Autodesk Inventor part; units mm, degrees
ref_plane "YZ Plane" through (0, 0, 0) normal (1, 0, 0) x (0, 1, 0)
ref_plane "XZ Plane" through (0, 0, 0) normal (0, 1, 0) x (-1, 0, 0)
ref_plane "XY Plane" through (0, 0, 0) normal (0, 0, 1) x (1, 0, 0)
ref_plane "Work Plane1" through (0, 0, 0) normal (0, 0, 1) x (1, 0, 0)
sketch "Sketch1" plane through (0, 0, 0) normal (0, 0, 1) x (1, 0, 0)
  circle A0 centre (0, 52.9) radius 8
  line L0 (-75, -117.1) -> (75, -117.1)
  line L1 (75, -117.1) -> (75, 82.9)
  line L2 (75, 82.9) -> (-75, 82.9)
  line L3 (-75, 82.9) -> (-75, -117.1)
  circle A1 centre (0, -87.1) radius 8
  circle A2 centre (0, -16.8) radius 16
  line L4 (0.031, -34.3) -> (-1.6246, -39.8894)
  line L5 (-1.6246, -39.8894) -> (-3.8779, -39.222)
  line L6 (-3.8779, -39.222) -> (-3.5087, -37.9755)
  line L7 (-3.5087, -37.9755) -> (-2.8854, -38.1601)
  line L8 (-2.8854, -38.1601) -> (-1.8914, -34.8042)
  line L9 (-1.8914, -34.8042) -> (-8.2196, -32.9297)
  line L10 (-8.2196, -32.9297) -> (-9.2136, -36.2856)
  line L11 (-9.2136, -36.2856) -> (-8.5904, -36.4702)
  line L12 (-8.5904, -36.4702) -> (-8.9843, -37.8)
  line L13 (-8.9843, -37.8) -> (-15.25, -37.8)
  line L14 (-15.25, -37.8) -> (-15.25, -39.8)
  line L15 (-15.25, -39.8) -> (-17.25, -39.8)
  line L16 (-17.25, -39.8) -> (-17.25, -37.8)
  arc A3 (-21, -34.05) -> (-17.25, -37.8) centre (-17.25, -34.05) ccw
  line L17 (-21, -34.05) -> (-23, -34.05)
  line L18 (-23, -34.05) -> (-23, -32.05)
  line L19 (-23, -32.05) -> (-21, -32.05)
  line L20 (-21, -32.05) -> (-21, -26.253)
  line L21 (-21, -26.253) -> (-19.5478, -25.71)
  arc A4 (-19.5478, -25.71) -> (-20.5984, -22.9) centre (-18.6632, -23.7779) ccw
  line L22 (-20.5984, -22.9) -> (-21.4365, -23.2134)
  line L23 (-21.4365, -23.2134) -> (-22.1807, -21.2229)
  line L24 (-22.1807, -21.2229) -> (-17.3057, -19.4003)
  arc A5 (-17.5, -16.831) -> (-17.3057, -19.4003) centre (0, -16.8) ccw
  line L25 (-17.5, -16.831) -> (-23.0894, -15.1754)
  line L26 (-23.0894, -15.1754) -> (-22.422, -12.9221)
  line L27 (-22.422, -12.9221) -> (-21.1755, -13.2913)
  line L28 (-21.1755, -13.2913) -> (-21.3601, -13.9146)
  line L29 (-21.3601, -13.9146) -> (-18.0042, -14.9086)
  line L30 (-18.0042, -14.9086) -> (-16.1297, -8.5804)
  line L31 (-16.1297, -8.5804) -> (-19.4856, -7.5864)
  line L32 (-19.4856, -7.5864) -> (-19.6702, -8.2096)
  line L33 (-19.6702, -8.2096) -> (-21, -7.8157)
  line L34 (-21, -7.8157) -> (-21, -1.55)
  line L35 (-21, -1.55) -> (-23, -1.55)
  line L36 (-23, -1.55) -> (-23, 0.45)
  line L37 (-23, 0.45) -> (-21, 0.45)
  arc A6 (-17.25, 4.2) -> (-21, 0.45) centre (-17.25, 0.45) ccw
  line L38 (-17.25, 4.2) -> (-17.25, 6.2)
  line L39 (-17.25, 6.2) -> (-15.25, 6.2)
  line L40 (-15.25, 6.2) -> (-15.25, 4.2)
  line L41 (-15.25, 4.2) -> (-9.453, 4.2)
  line L42 (-9.453, 4.2) -> (-8.91, 2.7478)
  arc A7 (-8.91, 2.7478) -> (-6.1, 3.7984) centre (-6.9779, 1.8632) ccw
  line L43 (-6.1, 3.7984) -> (-6.4134, 4.6365)
  line L44 (-6.4134, 4.6365) -> (-4.4229, 5.3807)
  line L45 (-4.4229, 5.3807) -> (-2.6003, 0.5057)
  arc A8 (-0.031, 0.7) -> (-2.6003, 0.5057) centre (0, -16.8) ccw
  line L46 (-0.031, 0.7) -> (1.6246, 6.2894)
  line L47 (1.6246, 6.2894) -> (3.8779, 5.622)
  line L48 (3.8779, 5.622) -> (3.5087, 4.3755)
  line L49 (3.5087, 4.3755) -> (2.8854, 4.5601)
  line L50 (2.8854, 4.5601) -> (1.8914, 1.2042)
  line L51 (1.8914, 1.2042) -> (8.2196, -0.6703)
  line L52 (8.2196, -0.6703) -> (9.2136, 2.6856)
  line L53 (9.2136, 2.6856) -> (8.5904, 2.8702)
  line L54 (8.5904, 2.8702) -> (8.9843, 4.2)
  line L55 (8.9843, 4.2) -> (15.25, 4.2)
  line L56 (15.25, 4.2) -> (15.25, 6.2)
  line L57 (15.25, 6.2) -> (17.25, 6.2)
  line L58 (17.25, 6.2) -> (17.25, 4.2)
  arc A9 (21, 0.45) -> (17.25, 4.2) centre (17.25, 0.45) ccw
  line L59 (21, 0.45) -> (23, 0.45)
  line L60 (23, 0.45) -> (23, -1.55)
  line L61 (23, -1.55) -> (21, -1.55)
  line L62 (21, -1.55) -> (21, -7.347)
  line L63 (21, -7.347) -> (19.5478, -7.89)
  arc A10 (19.5478, -7.89) -> (20.5984, -10.7) centre (18.6632, -9.8221) ccw
  line L64 (20.5984, -10.7) -> (21.4365, -10.3866)
  line L65 (21.4365, -10.3866) -> (22.1807, -12.3771)
  line L66 (22.1807, -12.3771) -> (17.3057, -14.1997)
  arc A11 (17.5, -16.769) -> (17.3057, -14.1997) centre (0, -16.8) ccw
  line L67 (17.5, -16.769) -> (23.0894, -18.4246)
  line L68 (23.0894, -18.4246) -> (22.422, -20.6779)
  line L69 (22.422, -20.6779) -> (21.1755, -20.3087)
  line L70 (21.1755, -20.3087) -> (21.3601, -19.6854)
  line L71 (21.3601, -19.6854) -> (18.0042, -18.6914)
  line L72 (18.0042, -18.6914) -> (16.1297, -25.0196)
  line L73 (16.1297, -25.0196) -> (19.4856, -26.0136)
  line L74 (19.4856, -26.0136) -> (19.6702, -25.3904)
  line L75 (19.6702, -25.3904) -> (21, -25.7843)
  line L76 (21, -25.7843) -> (21, -32.05)
  line L77 (21, -32.05) -> (23, -32.05)
  line L78 (23, -32.05) -> (23, -34.05)
  line L79 (23, -34.05) -> (21, -34.05)
  arc A12 (17.25, -37.8) -> (21, -34.05) centre (17.25, -34.05) ccw
  line L80 (17.25, -37.8) -> (17.25, -39.8)
  line L81 (17.25, -39.8) -> (15.25, -39.8)
  line L82 (15.25, -39.8) -> (15.25, -37.8)
  line L83 (15.25, -37.8) -> (9.453, -37.8)
  line L84 (9.453, -37.8) -> (8.91, -36.3478)
  arc A13 (8.91, -36.3478) -> (6.1, -37.3984) centre (6.9779, -35.4632) ccw
  line L85 (6.1, -37.3984) -> (6.4134, -38.2365)
  line L86 (6.4134, -38.2365) -> (4.4229, -38.9807)
  line L87 (4.4229, -38.9807) -> (2.6003, -34.1057)
  arc A14 (0.031, -34.3) -> (2.6003, -34.1057) centre (0, -16.8) ccw
extrude "Extrusion1" add sketch "Sketch1" along normal blind 20 contours L3 L2 L1 L0
properties part number "Soporte Pistón"
The model under review builds one solid part; all positions refer to its coordinate system, in mm. Coordinates: 2 decimals unless noted, no trailing zeros. Write each loop counter-clockwise with the first axis right and the second up, starting at its lowest first coordinate (ties: lowest second). Pieces come first, ordered by that corner, then holes.
1) To check wall thickness, follow probe 1 along X at (y, z) = (2.5, 7.5); probe 2 along Y at (x, z) = (7, 8); probe 3 along X at (y, z) = (-94.5, 9.5). State the ranges of each line that lie inside material, in increasing order.
2) We need section B-B on z = 7.75. Count the separate pieces of the cut face and the enclosed holes in it, then the cut area to 3 significant figures.
3) The part is to be moulded in two halves that separate along Y. For faces 1 (the face through (-75, -16, 10)), 2 (the face through (-12, 4.2, 10)), say which applies: pulls with the +Y half, pulls with the -Y half, needs draft (parallel to the pull), parting line crosses it, or undercut.
4) We need section A-A on y = 52.9. State the section outline as (x, z) points.
Answer list:
1. probe 1: x = -75 to -20.39, -9.01 to -4.95, -3.35 to 0.5, 2.28 to 9.16, 20.39 to 75
1. probe 2: y = -117.1 to -90.97, -83.23 to -33.34, -0.31 to 49.03, 56.77 to 82.9
1. probe 3: x = -75 to -3.04, 3.04 to 75
2. separate pieces: 1
2. enclosed holes: 3
2. area: 28,000 mm2
3. face 1: needs draft
3. face 2: undercut
4. outline: (-75, 0) - (-8, 0) - (-8, 20) - (-75, 20) - close; (8, 0) - (75, 0) - (75, 20) - (8, 20) - close
